For this review, take the finished solid that the model builds, in its own axes (mm). Give positions to 0.01 mm unless a question says otherwise; leave off trailing zeros. Loops run counter-clockwise (first coordinate to the right, second up) from the corner with the lowest first, then second, coordinate; pieces in that order, holes last.
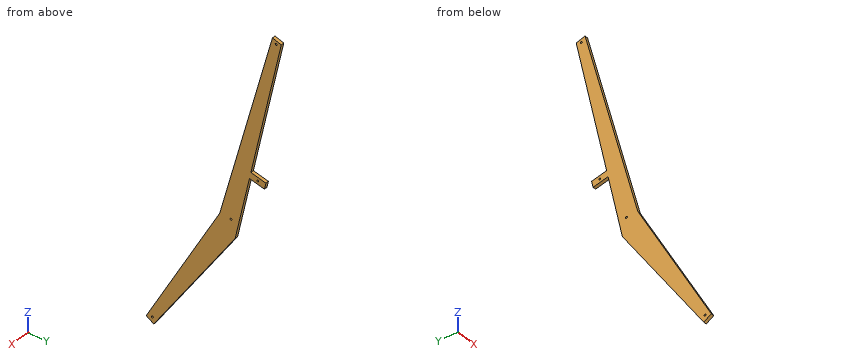
```python
from build123d import *

# Parameters (mm, degrees)
SKETCH_1_R          = 0.6
EXTRUDE_1_DEPTH     = 2
SKETCH_2_W          = 2
SKETCH_2_H          = 4.371689855
EXTRUDE_2_DEPTH     = 10
SKETCH_3_R          = 0.6
CUT_EXTRUDE_1_DEPTH = 139.866853183


with BuildPart() as part:
    # 草图1 → 凸台-拉伸1 (new body)
    with BuildSketch(Plane(origin=(0, 0, 0), x_dir=(0, 0, -1), z_dir=(1, 0, 0))):
        Polygon((-125.665306235, 32.633935399), (10.915414504, 2.625615762), (89.98290861, -50.249012451), (87.007289875, -55.156822928), (-0.286231168, -7.394028573), (-127.427343209, 26.898499434), align=None)
        Circle(SKETCH_1_R, mode=Mode.SUBTRACT)
        with Locations((85.929781066, -51.147558357)):
            Circle(SKETCH_1_R, mode=Mode.SUBTRACT)
        with Locations((-124.4283455, 29.268026496)):
            Circle(SKETCH_1_R, mode=Mode.SUBTRACT)
    extrude(amount=EXTRUDE_1_DEPTH)

    # 草图2 → 凸台-拉伸2 (add)
    with BuildSketch(Plane(origin=(0, 4.792506233, -1.052967491), x_dir=(1, 0, 0), z_dir=(0, 0.9767036122693339, -0.21459276264598237))):
        with Locations((1, -35.420952271)):
            Rectangle(SKETCH_2_W, SKETCH_2_H)
    extrude(amount=EXTRUDE_2_DEPTH)

    # 草图3 → 切除-拉伸1 (cut, through all)
    with BuildSketch(Plane(origin=(2, 0, 0), x_dir=(0, 0, -1), z_dir=(1, 0, 0))):
        with Locations((-32.469840729, 17.277104298)):
            Circle(SKETCH_3_R)
    extrude(amount=-CUT_EXTRUDE_1_DEPTH, mode=Mode.SUBTRACT)


solid = part.part
```
Item 1: Take a section at A-A on x = 0.7. Give the boundary of the cut face in (y, z), and give its area (3 significant figures).
Answer:
outline: (-55.16, -87.01) - (-50.25, -89.98) - (2.63, -10.92) - (11.92, 31.41) - (21.69, 29.26) - (22.63, 33.53) - (12.86, 35.68) - (32.63, 125.67) - (26.9, 127.43) - (-7.39, 0.29) - close; hole circle Ø1.2 at (-51.15, -85.93); hole circle Ø1.2 at (0, 0); hole circle Ø1.2 at (17.28, 32.47); hole circle Ø1.2 at (29.27, 124.43)
area: 2,260 mm2
Item 2: For L1, parallel to Y at x = 0.4, z = 0; L2, parallel to Y at x = 1.3, z = 20; L3, parallel to Y at x = 0.9, z = 94, list the stretches that pass through material, from the lowest coordinate up.
Answer:
L1: y = -7.55 to -0.6, 0.6 to 5.02
L2: y = -2.08 to 9.42
L3: y = 17.88 to 25.68
Item 3: Take a section at C-C on z = 73. Give the boundary of the cut face in (x, y), and give its area (3 significant figures).
Answer:
outline: (0, 12.22) - (2, 12.22) - (2, 21.06) - (0, 21.06) - close
area: 17.7 mm2
Item 4: Take a section at B-B on y = -10. Give the boundary of the cut face in (x, z).
Answer:
outline: (0, -29.8) - (2, -29.8) - (2, -4.48) - (0, -4.48) - close
